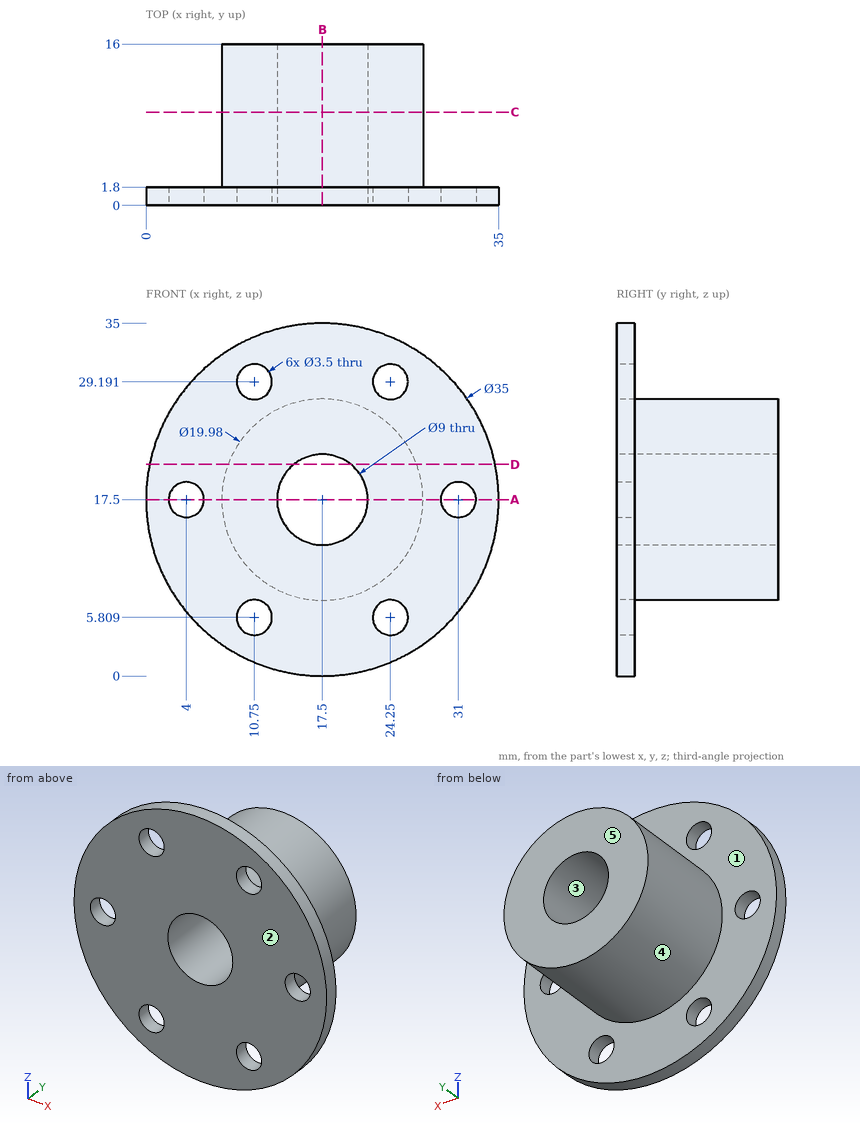
Verification items for this drawing (mm, ordinates from the low corner). A direction names the side the tool comes from. Round coordinates to 2 decimals unless told otherwise and drop trailing zeros. Loops run counter-clockwise (first coordinate to the right, second up) from the corner with the lowest first, then second, coordinate; pieces in that order, holes last. Notation, with made-up numbers: (-38.5, 85) -> (-24.5, 85) arc R27 ccw to (-24.5, 114) -> close; hole circle Ø11 at (40.25, 54.25). An arc over 180 degrees is marked (long way). Write item = value, one per line. Start each with the question number.
1) Release check for a two-part mould opening along X. For the marked faces 3, 4 and 5 record: released by +X, released by -X, zero draft, split by the parting line, or undercut.
2) Sectioned sample at A-A, the plane z = 17.5. Record the cut outline in (x, y).
3) Sectioned sample at D-D, the plane z = 21. Record the cut outline in (x, y).
4) Sectioned sample at C-C, the plane y = 9.25. Record the cut outline in (x, z), plus the area to 3 significant figures.
5) Thickness scan on probe 1 along X at (y, z) = (4, 17.5); probe 2 along X at (y, z) = (1.75, 28.5); probe 3 along Y at (x, z) = (6.5, 26.5). Record the ranges inside material, lowest first.
6) Sectioned sample at B-B, the plane x = 17.5. Record the cut outline in (y, z).
7) Gauge pin test, flat ends, axial feed: pin 1 Ø5 at (x, y) = (14.5, 14) entering from -Z; pin 2 Ø1 at (y, z) = (12.5, 17) entering from -X; pin 3 Ø3 at (y, z) = (7.5, 16.5) entering from +X; pin 4 Ø2 at (x, z) = (4, 17.5) entering from -Y. Record the tip position at first contact, or that the pin passes through.
8) Set-up check for the marked faces 1 and 2: record each of +Z, -Z, +X, -X, +Y, -Y from which the full face is reachable in a straight line by a thin tool's end or side.
Results are:
q1.face_3 = undercut
q1.face_4 = split by the parting line
q1.face_5 = zero draft
q2.outline = (0, 0) -> (2.25, 0) -> (2.25, 1.8) -> (0, 1.8) -> close; (5.75, 0) -> (13, 0) -> (13, 16) -> (7.51, 16) -> (7.51, 1.8) -> (5.75, 1.8) -> close; (22, 0) -> (29.25, 0) -> (29.25, 1.8) -> (27.49, 1.8) -> (27.49, 16) -> (22, 16) -> close; (32.75, 0) -> (35, 0) -> (35, 1.8) -> (32.75, 1.8) -> close
q3.outline = (0.35, 0) -> (14.67, 0) -> (14.67, 16) -> (8.14, 16) -> (8.14, 1.8) -> (0.35, 1.8) -> close; (20.33, 0) -> (34.65, 0) -> (34.65, 1.8) -> (26.86, 1.8) -> (26.86, 16) -> (20.33, 16) -> close
q4.outline = circle Ø19.98 at (17.5, 17.5); hole circle Ø9 at (17.5, 17.5)
q4.area = 250 mm^2
q5.probe_1 = 7.51 to 13, 22 to 27.49
q5.probe_2 = 3.89 to 9.14, 12.36 to 22.64, 25.86 to 31.11
q5.probe_3 = 0 to 1.8
q6.outline = (0, 0) -> (1.8, 0) -> (1.8, 7.51) -> (16, 7.51) -> (16, 13) -> (0, 13) -> close; (0, 22) -> (16, 22) -> (16, 27.49) -> (1.8, 27.49) -> (1.8, 35) -> (0, 35) -> close
q7.pin_1 = 7.52
q7.pin_2 = 7.51
q7.pin_3 = 27.49
q7.pin_4 = through
q8.face_1 = +Y
q8.face_2 = +Z, -Z, +X, -X, -Y
